Model file for the job. Use its own axes, mm. A direction names the side the tool comes from. Coordinates: 2 decimals unless noted, no trailing zeros. Order: outer loops, then holes, each group sorted by start corner. A loop starts at its lowest first (then second) coordinate and runs counter-clockwise, first axis right, second up.
from build123d import *

# Parameters (mm, degrees)
BOSS_EXTRUDE1_DEPTH = 19.05
SKETCH2_W           = 12.7
SKETCH2_H           = 12.7
CUT_EXTRUDE1_DEPTH  = 272.852903886
SKETCH3_R           = 2.413
CUT_EXTRUDE2_DEPTH  = 354.991519469


with BuildPart() as part:
    # Sketch1 → Boss-Extrude1 (new body)
    with BuildSketch(Plane(origin=(0, 0, 0), x_dir=(0, 0, -1), z_dir=(1, 0, 0))):
        Polygon((268.494858146, -191.807817407), (268.494858146, -229.907817407), (249.444858146, -229.907817407), (249.444858146, -198.74145037), align=None)
    extrude(amount=BOSS_EXTRUDE1_DEPTH)

    # Sketch2 → Cut-Extrude1 (cut, through all)
    with BuildSketch(Plane.XZ.offset(229.907817407)):
        with Locations((9.525, -258.969858146)):
            Rectangle(SKETCH2_W, SKETCH2_H)
    extrude(amount=-CUT_EXTRUDE1_DEPTH, mode=Mode.SUBTRACT)

    # Sketch3 → Cut-Extrude2 (cut, through all)
    with BuildSketch(Plane(origin=(19.05, 0, 0), x_dir=(0, 0, -1), z_dir=(1, 0, 0))):
        with Locations((258.969858146, -217.207817407)):
            Circle(SKETCH3_R)
    extrude(amount=-CUT_EXTRUDE2_DEPTH, mode=Mode.SUBTRACT)


solid = part.part
Q1. Cut at C-C, the plane z = -254. List the corners of the cut face in (x, y) (3 decimals).
Established:
outline: (0, -229.908) - (3.175, -229.908) - (3.175, -197.084) - (0, -197.084) - close; (15.875, -229.908) - (19.05, -229.908) - (19.05, -197.084) - (15.875, -197.084) - close
Q2. Cut at B-B, the plane y = -226. List the corners of the cut face in (x, z) (3 decimals), plus the area to 3 significant figures.
Established:
outline: (0, -268.495) - (19.05, -268.495) - (19.05, -249.445) - (0, -249.445) - close; hole (3.175, -265.32) - (15.875, -265.32) - (15.875, -252.62) - (3.175, -252.62) - close
area: 202 mm2
Q3. Mould opens along Z. For faces 1 (the face through (9, -211, -268.495)), 2 (the face through (3, -196.1, -256.7)), 3 (the face through (9, -214, -252.62)), 4 (the face through (1.61, -215.58, -257.19)) say: pulls with the +Z half, pulls with the -Z half, needs draft (parallel to the pull), parting line crosses it, or undercut.
Established:
face 1: pulls with the -Z half
face 2: pulls with the +Z half
face 3: undercut
face 4: undercut
Q4. Probe line 1 (Z direction, x = 5.5, y = -207); line 2 (X direction, y = -195, z = -260.5) (3 decimals); line 3 (Y direction, x = 2.25, z = -252). List the from-to ranges inside material, lowest first.
Established:
line 1: z = -268.49 to -265.32, -252.62 to -249.44
line 2: x = 0 to 3.175, 15.875 to 19.05
line 3: y = -229.91 to -197.81
Q5. Which spindle directions (+Z, -Z, +X, -X, +Y, -Y) get a long thin tool onto all of the face, cutting with end or side? Do faces 5 (the face through (9, -212, -265.32)), 6 (the face through (0, -211, -259)). Say none if no direction does.
Established:
face 5: +Y, -Y
face 6: +Z, -Z, -X, +Y, -Y
Q6. Cut at D-D, the plane y = -216. List the corners of the cut face in (x, z) (3 decimals).
Established:
outline: (0, -268.495) - (19.05, -268.495) - (19.05, -261.059) - (15.875, -261.059) - (15.875, -265.32) - (3.175, -265.32) - (3.175, -261.059) - (0, -261.059) - close; (0, -256.881) - (3.175, -256.881) - (3.175, -252.62) - (15.875, -252.62) - (15.875, -256.881) - (19.05, -256.881) - (19.05, -249.445) - (0, -249.445) - close
Q7. Cut at A-A, the plane x = 8.75. List the corners of the cut face in (y, z).
Established:
outline: (-229.91, -268.49) - (-191.81, -268.49) - (-192.96, -265.32) - (-229.91, -265.32) - close; (-229.91, -252.62) - (-197.59, -252.62) - (-198.74, -249.44) - (-229.91, -249.44) - close
Q8. Drop flat-ended pins along their axis: P1, Ø3, axis at y = -217.21, z = -258.97, coming from the +X side; P2, Ø10, axis at x = 10.5, z = -264, coming from the +Y side; P3, Ø4, axis at y = -207.5, z = -253, coming from the -X side. Give the stop position or say it passes through.
Established:
P1: passes through
P2: stops at y = -191.81
P3: stops at x = 0
